Print and shaded views of the part. All mm, measured from the part's lowest x, y and z. A direction names the side the tool comes from. Coordinates: 2 decimals unless noted, no trailing zeros. Write each loop counter-clockwise with the first axis right and the second up, starting at its lowest first coordinate (ties: lowest second). Pieces come first, ordered by that corner, then holes. Notation, with made-up numbers: (21.25, 16) -> (59.25, 16) arc R19 cw to (59.25, 28) -> close; hole circle Ø2 at (22.5, 64.25). An arc over 180 degrees is marked (long way). Write item = value, one per line.
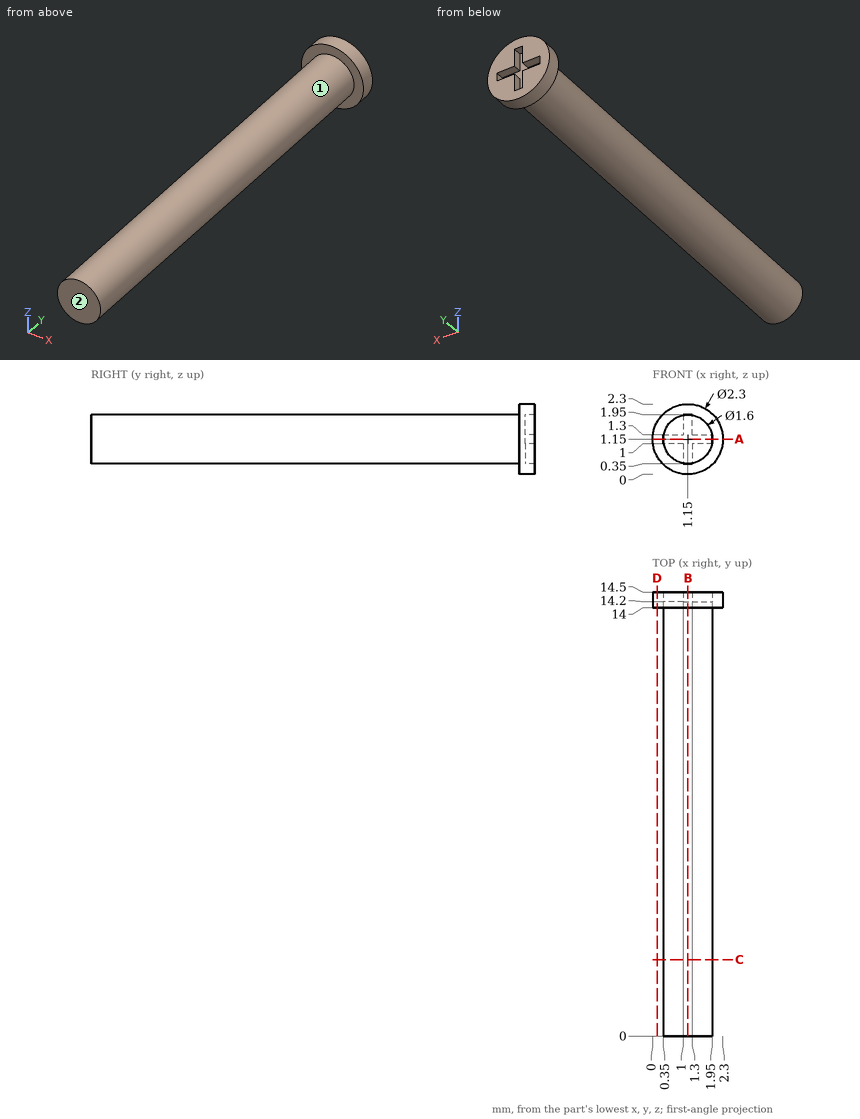
Q1. Which spindle directions (+Z, -Z, +X, -X, +Y, -Y) get a long thin tool onto all of the face, cutting with end or side? Do the marked faces 1 and 2. Say none if no direction does.
Model answer:
face_1 = -Y
face_2 = +Z, -Z, +X, -X, -Y
Q2. Saw through at A-A on z = 1.15. Give the cut face in (x, y).
Model answer:
outline = (0, 14) -> (0.35, 14) -> (0.35, 0) -> (1.95, 0) -> (1.95, 14) -> (2.3, 14) -> (2.3, 14.5) -> (1.95, 14.5) -> (1.95, 14.2) -> (0.35, 14.2) -> (0.35, 14.5) -> (0, 14.5) -> close
Q3. Probe line 1 (Y direction, x = 0.35, z = 1.8); line 2 (Y direction, x = 1.05, z = 0.5); line 3 (X direction, y = 9.5, z = 1.1). List the from-to ranges inside material, lowest first. Write a range as from..to.
Model answer:
line_1 = 14..14.5
line_2 = 0..14.2
line_3 = 0.35..1.95
Q4. Saw through at D-D on x = 0.15. Give the cut face in (y, z).
Model answer:
outline = (14, 0.58) -> (14.5, 0.58) -> (14.5, 1.72) -> (14, 1.72) -> close
Q5. Saw through at C-C on y = 2.5. Give the cut face in (x, z), and give its area (3 significant figures).
Model answer:
outline = circle Ø1.6 at (1.15, 1.15)
area = 2.01 mm²
Q6. Pin check, flat tip, straight feed: pin 1 (1 mm diameter, centred on x = 1, y = 6, fed in from -Z). Stop position of the tip, or through.
Model answer:
pin_1 = 0.35
Q7. Saw through at B-B on x = 1.15. Give the cut face in (y, z).
Model answer:
outline = (0, 0.35) -> (14, 0.35) -> (14, 0) -> (14.5, 0) -> (14.5, 0.35) -> (14.2, 0.35) -> (14.2, 1.95) -> (14.5, 1.95) -> (14.5, 2.3) -> (14, 2.3) -> (14, 1.95) -> (0, 1.95) -> close
